```python
from build123d import *

# Parameters (mm, degrees)
BOSS_EXTRUDE1_DEPTH = 2
SKETCH2_R           = 1.55
CUT_EXTRUDE1_DEPTH  = 5
SKETCH3_W           = 12
SKETCH3_H           = 8
CUT_EXTRUDE2_DEPTH  = 5
SKETCH4_R           = 1.5
CUT_EXTRUDE4_DEPTH  = 10


with BuildPart() as part:
    # Sketch1 → Boss-Extrude1 (new body, symmetric)
    with BuildSketch(Plane(origin=(0, 0, 0), x_dir=(1, 0, 0), z_dir=(0, 1, 0))):
        with BuildLine():
            ThreePointArc((-6, 79.774682701), (0, -80), (6, 79.774682701))
            ThreePointArc((6, 79.774682701), (0, 80), (-6, 79.774682701))
        make_face()
    extrude(amount=BOSS_EXTRUDE1_DEPTH, both=True)

    # Sketch2 → Cut-Extrude1 (cut, through all)
    with BuildSketch(Plane.XZ.offset(2)):
        with Locations((75, 0)):
            Circle(SKETCH2_R)
        with Locations((-75, 0)):
            Circle(SKETCH2_R)
    extrude(amount=-CUT_EXTRUDE1_DEPTH, mode=Mode.SUBTRACT)

    # Sketch3 → Cut-Extrude2 (cut, through all)
    with BuildSketch(Plane(origin=(0, 2, 0), x_dir=(1, 0, 0), z_dir=(0, 1, 0))):
        Polygon((43.765371804, 32.196152423), (49.765371804, 21.803847577), (42.837168574, 17.803847577), (36.837168574, 28.196152423), align=None)
        with Locations((0, 50)):
            Rectangle(SKETCH3_W, SKETCH3_H)
        Polygon((49.765371804, -21.803847577), (43.765371804, -32.196152423), (36.837168574, -28.196152423), (42.837168574, -17.803847577), align=None)
        with Locations((0, -50)):
            Rectangle(SKETCH3_W, SKETCH3_H)
        Polygon((-43.765371804, -32.196152423), (-49.765371804, -21.803847577), (-42.837168574, -17.803847577), (-36.837168574, -28.196152423), align=None)
        Polygon((-49.765371804, 21.803847577), (-43.765371804, 32.196152423), (-36.837168574, 28.196152423), (-42.837168574, 17.803847577), align=None)
    extrude(amount=-CUT_EXTRUDE2_DEPTH, mode=Mode.SUBTRACT)

    # Sketch4 → Cut-Extrude4 (cut)
    with BuildSketch(Plane(origin=(0, 2, 0), x_dir=(1, 0, 0), z_dir=(0, 1, 0))):
        with Locations((0, -29.5)):
            Circle(SKETCH4_R)
        with Locations((-25.547749412, 14.75)):
            Circle(SKETCH4_R)
        with Locations((-25.547749412, -14.75)):
            Circle(SKETCH4_R)
        with Locations((25.547749412, -14.75)):
            Circle(SKETCH4_R)
        with Locations((25.547749412, 14.75)):
            Circle(SKETCH4_R)
        with Locations((0, 29.5)):
            Circle(SKETCH4_R)
    extrude(amount=-CUT_EXTRUDE4_DEPTH, mode=Mode.SUBTRACT)


solid = part.part
```
Geometry: final body of the model. Coordinates: model frame, mm. Coordinates: 2 decimals unless noted, no trailing zeros. Order: outer loops, then holes, each group sorted by start corner. A loop starts at its lowest first (then second) coordinate and runs counter-clockwise, first axis right, second up. Notation, with made-up numbers: (-38, -19) -> (-14, -19) arc R25 cw to (-14, -2) -> close; hole circle Ø6 at (-3.75, 60). An arc over 180 degrees is marked (long way). Use CSV: the item, a comma, the result in double quotes.
1) Section A-A on y = -0.65. State how many separate pieces and enclosed holes the cut face has, then the cut area to 3 significant figures.
Findings:
separate pieces,"1"
enclosed holes,"14"
area,"19,500 mm^2"
2) Pin query (flat end, axial travel): pin 1 Ø1 at (x, y) = (-56, -1.5) entering from -Z; pin 2 Ø1.5 at (x, y) = (-17.5, 1) entering from +Z; pin 3 Ø2 at (y, z) = (0.5, -48.5) entering from +X. Return the tip coordinate at first contact, or that it passes through.
Findings:
pin 1,"stops at z = -57.62"
pin 2,"stops at z = 78.23"
pin 3,"stops at x = 64.37"
3) Mould query, pull axis Z, two halves, no side actions, for faces 1 (the flat face through (-1, -2, -1)), 2 (the flat face through (40.253, 0.028, -30.168)). Classes: +Z half, -Z half, draft (parallel to the pull), parting line (faces both ways), or undercut.
Findings:
face 1,"draft"
face 2,"undercut"
4) Line query: line 1 (Z direction, x = 0, y = -1.7); line 2 (X direction, y = -0.6, z = -29.5); line 3 (Z direction, x = 43, y = 1.7). Output: solid intervals per line, ascending.
Findings:
line 1,"z = -80 to -54, -46 to -31, -28 to 28, 31 to 46, 54 to 80"
line 2,"x = -74.36 to -45.32, -39.1 to -1.5, 1.5 to 39.1, 45.32 to 74.36"
line 3,"z = -67.46 to -31.75, -17.9 to 17.9, 31.75 to 67.46"
5) Section C-C on x = 66. Output: boundary loops of the cut face in (y, z), then the cut area to 3 significant figures.
Findings:
outline,"(-2, -45.21) -> (2, -45.21) -> (2, 45.21) -> (-2, 45.21) -> close"
area,"362 mm^2"
6) Section B-B on z = 68. Output: boundary loops of the cut face in (x, y).
Findings:
outline,"(-42.14, -2) -> (42.14, -2) -> (42.14, 2) -> (-42.14, 2) -> close"
